```python
from build123d import *

# Parameters (mm, degrees)
SKETCH1_W           = 200
SKETCH1_H           = 115
SKETCH1_R           = 38.5
SKETCH1_R_2         = 2
SKETCH1_R_3         = 1.5
SKETCH1_W_2         = 27.5
SKETCH1_H_2         = 20
SKETCH1_W_3         = 14
SKETCH1_H_3         = 15
BOSS_EXTRUDE1_DEPTH = 5


with BuildPart() as part:
    # Sketch1 → Boss-Extrude1 (new body)
    with BuildSketch(Plane.XY):
        Rectangle(SKETCH1_W, SKETCH1_H)
        with Locations((-34.5, 7)):
            Circle(SKETCH1_R, mode=Mode.SUBTRACT)
        with Locations((-70, 42.5)):
            Circle(SKETCH1_R_2, mode=Mode.SUBTRACT)
        with Locations((1, 42.5)):
            Circle(SKETCH1_R_2, mode=Mode.SUBTRACT)
        with Locations((1, -28.5)):
            Circle(SKETCH1_R_2, mode=Mode.SUBTRACT)
        with Locations((-70, -28.5)):
            Circle(SKETCH1_R_2, mode=Mode.SUBTRACT)
        with Locations((71.25, 34.5)):
            Circle(SKETCH1_R_3, mode=Mode.SUBTRACT)
        with Locations(Location((31.25, 34.5, 0), (0, 0, 180))):
            Circle(SKETCH1_R_3, mode=Mode.SUBTRACT)
        with Locations((51.25, 34.5)):
            Rectangle(SKETCH1_W_2, SKETCH1_H_2, mode=Mode.SUBTRACT)
        with Locations((51.25, 4.5)):
            Rectangle(SKETCH1_W_3, SKETCH1_H_3, mode=Mode.SUBTRACT)
    extrude(amount=BOSS_EXTRUDE1_DEPTH)


solid = part.part
```
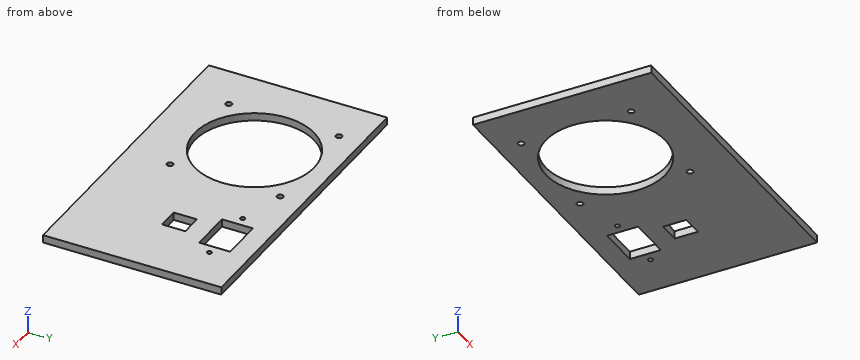
The listing builds one solid part. Answer for the finished solid, in the listing's coordinates (mm). Give positions to 0.01 mm unless a question says otherwise; leave off trailing zeros. Order: outer loops, then holes, each group sorted by start corner. A loop starts at its lowest first (then second) coordinate and runs counter-clockwise, first axis right, second up. Notation, with made-up numbers: (7, 3.5) -> (27, 3.5) arc R15 cw to (27, 10.5) -> close; hole circle Ø7 at (40.25, 55.25). An arc over 180 degrees is marked (long way). Answer as a JSON object with one key per item and string values. Group by question number.
Item 1: Consider L1, parallel to Y at x = 53.5, z = 0.85; L2, parallel to Y at x = -70, z = 2.2; L3, parallel to X at y = 28.5, z = 0.9. Determine where each line is inside the solid, lowest interval first. Write a range as from..to.
Item 2: The part is cut by section C-C on y = -28.5. Write down the section's boundary in (x, z).
Item 3: The part is cut by section B-B on x = -34.5. Write down the section's boundary in (y, z).
Item 4: The part is cut by section D-D on x = 1. Write down the section's boundary in (y, z), and give its area (3 significant figures).
Item 5: The part is cut by section A-A on z = 3.6. Give the number of separate pieces and of enclosed holes in the cut face, and give its area (3 significant figures).
Result set:
{
 "1": {"L1": "-57.5..-3, 12..24.5, 44.5..57.5", "L2": "-57.5..-30.5, -26.5..-7.9, 21.9..40.5, 44.5..57.5", "L3": "-100..-66.44, -2.56..37.5, 65..100"},
 "2": {"outline": "(-100, 0) -> (-72, 0) -> (-72, 5) -> (-100, 5) -> close; (-68, 0) -> (-49.4, 0) -> (-49.4, 5) -> (-68, 5) -> close; (-19.6, 0) -> (-1, 0) -> (-1, 5) -> (-19.6, 5) -> close; (3, 0) -> (100, 0) -> (100, 5) -> (3, 5) -> close"},
 "3": {"outline": "(-57.5, 0) -> (-31.5, 0) -> (-31.5, 5) -> (-57.5, 5) -> close; (45.5, 0) -> (57.5, 0) -> (57.5, 5) -> (45.5, 5) -> close"},
 "4": {"outline": "(-57.5, 0) -> (-30.5, 0) -> (-30.5, 5) -> (-57.5, 5) -> close; (-26.5, 0) -> (-7.9, 0) -> (-7.9, 5) -> (-26.5, 5) -> close; (21.9, 0) -> (40.5, 0) -> (40.5, 5) -> (21.9, 5) -> close; (44.5, 0) -> (57.5, 0) -> (57.5, 5) -> (44.5, 5) -> close", "area": "386 mm²"},
 "5": {"separate pieces": "1", "enclosed holes": "9", "area": "17,500 mm²"}
}
